```python
from build123d import *

# Parameters (mm, degrees)
F0_R      = 18
F0_R_2    = 5.95
F1_DEPTH  = 4
F2_R      = 18
F2_R_2    = 16
F3_DEPTH  = 1.5
F5_DEPTH  = 1.5
F6_SIZE   = 0.3
F7_COUNT  = 3
F8_R      = 0.75
F9_DEPTH  = 2.5
F10_COUNT = 6
F11_R     = 17
F12_DEPTH = 0.5
F13_SIZE  = 1


with BuildPart() as f1:
    # F0 (on Top) → F1 (new body)
    with BuildSketch(Plane.XY):
        Circle(F0_R)
        Circle(F0_R_2, mode=Mode.SUBTRACT)
    extrude(amount=-F1_DEPTH)

    # F2 (on Top) → F3 (join)
    with BuildSketch(Plane.XY):
        Circle(F2_R)
        Circle(F2_R_2, mode=Mode.SUBTRACT)
    extrude(amount=F3_DEPTH)

    # F4 (on Top) → F5 (join)
    with BuildSketch(Plane.XY):
        with BuildLine():
            Line((-1, -16.7781973636), (1, -16.7781973636))
            Line((1, -16.7781973636), (1, -3.8729833462))
            ThreePointArc((1, -3.8729833462), (0, -4), (-1, -3.8729833462))
            Line((-1, -3.8729833462), (-1, -16.7781973636))
        make_face()
        with BuildLine():
            ThreePointArc((-1, -3.8729833462), (0, -4), (1, -3.8729833462))
            Line((1, -3.8729833462), (1, 3.8729833462))
            ThreePointArc((1, 3.8729833462), (0, 4), (-1, 3.8729833462))
            Line((-1, 3.8729833462), (-1, -3.8729833462))
        make_face()
        with BuildLine():
            Line((1, 3.8729833462), (1, -3.8729833462))
            ThreePointArc((1, -3.8729833462), (3.1622776602, -2.4494897428), (4, 0))
            ThreePointArc((4, 0), (3.1622776602, 2.4494897428), (1, 3.8729833462))
        make_face()
        with BuildLine():
            ThreePointArc((-1, 3.8729833462), (-4, 0), (-1, -3.8729833462))
            Line((-1, -3.8729833462), (-1, 3.8729833462))
        make_face()
        with BuildLine():
            ThreePointArc((-1, 3.8729833462), (0, 4), (1, 3.8729833462))
            Line((1, 3.8729833462), (1, 16.7781973636))
            Line((1, 16.7781973636), (-1, 16.7781973636))
            Line((-1, 16.7781973636), (-1, 3.8729833462))
        make_face()
    extrude(amount=F5_DEPTH)

    # F6
    f6_edges = [f1.edges().sort_by_distance(p)[0] for p in [
        (-18, 0, 1.5),
        (16, 0, 1.5),
        (1, -9.920851, 1.5),
        (4, 0, 1.5),
        (1, 9.920851, 1.5),
        (-16, 0, 1.5),
        (-1, 9.920851, 1.5),
        (-4, 0, 1.5),
        (-1, -9.920851, 1.5),
    ]]
    chamfer(f6_edges, length=F6_SIZE)

    # F7: F1 ×3 about axis
    f7_axis = Axis((0, 0, 0), (0, 0, 1))


with BuildPart() as f1_1:
    add(f1.part)
    for i in range(1, F7_COUNT):
        add(f1.part.rotate(f7_axis, i * 360 / F7_COUNT))

    # F8 (on Top) → F9 (join)
    with BuildSketch(Plane.XY):
        with Locations((0, -16.8108288199)):
            Circle(F8_R)
    extrude(amount=F9_DEPTH)

    # F10: F1 ×6 about axis
    f10_axis = Axis((0, 0, 1.2), (0, 0, -1))


with BuildPart() as f1_2:
    add(f1_1.part)
    for i in range(1, F10_COUNT):
        add(f1_1.part.rotate(f10_axis, i * 360 / F10_COUNT))

    # F11 (on Top) → F12 (join)
    with BuildSketch(Plane.XY):
        Circle(F11_R)
    extrude(amount=F12_DEPTH)

    # F13
    f13_edges = [f1_2.edges().sort_by_distance(p)[0] for p in [
        (-5.95, 0, 0),
    ]]
    chamfer(f13_edges, length=F13_SIZE)


solid = f1_2.part
```
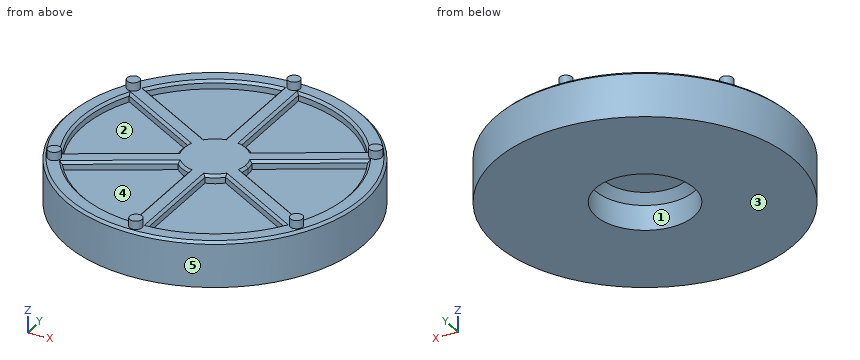
Input: part model. Units: mm. Frame: model coordinates. Face numbers are marked on the shaded views. A direction names the side the tool comes from. Give positions to 0.01 mm unless a question says otherwise; leave off trailing zeros. Write each loop counter-clockwise with the first axis right and the second up, starting at its lowest first coordinate (ties: lowest second). Pieces come first, ordered by that corner, then holes. Notation, with made-up numbers: (18, 85) - (36, 85) arc R13 cw to (36, 95) - close; hole circle Ø2 at (39.25, 83.25). An arc over 180 degrees is marked (long way). Write item = value, one per line. Start each with the question number.
1) Draft query along X for the marked faces 3, 4 and 5. Return one class per face: pulls with the +X half, pulls with the -X half, needs draft (parallel to the pull), parting line crosses it, or undercut.
2) Cut plane A-A (x = 0). Return loops of the section in (y, z).
3) Pin query (flat end, axial travel): pin 1 (3 mm diameter, centred on x = -1.5, y = 1, fed in from -Z); pin 2 (10 mm diameter, centred on x = 4.5, y = 7.5, fed in from +Z); pin 3 (3 mm diameter, centred on y = -6, z = -1, fed in from -X). Return the tip coordinate at first contact, or that it passes through.
4) Material intervals for L1, parallel to Y at x = 0, z = -3.25; L2, parallel to X at y = 3, z = 0.75; L3, parallel to Z at x = 8.5, y = -10, sorted ascending. Write a range as [from, to].
5) Cut plane B-B (z = -1.5). Return loops of the section in (x, y), and give its area (3 significant figures).
6) Reachability of the marked faces 1 and 2 from +Z, -Z, +X, -X, +Y, -Y: full face, straight path, thin tool, end or side. Return the list, or none.
Answers follow:
q1.face_3 = needs draft
q1.face_4 = undercut
q1.face_5 = parting line crosses it
q2.outline = (-18, -4) - (-5.95, -4) - (-5.95, -1) - (-4.95, 0) - (4.95, 0) - (5.95, -1) - (5.95, -4) - (18, -4) - (18, 1.2) - (17.7, 1.5) - (17.56, 1.5) - (17.56, 2.5) - (16.06, 2.5) - (16.06, 1.5) - (-16.06, 1.5) - (-16.06, 2.5) - (-17.56, 2.5) - (-17.56, 1.5) - (-17.7, 1.5) - (-18, 1.2) - close
q3.pin_1 = 0
q3.pin_2 = 1.5
q3.pin_3 = -17.43
q4.L1 = [-18, -5.95], [5.95, 18]
q4.L2 = [-17.75, -15.72], [-7.2, -3.2], [-2.65, 2.65], [3.2, 7.2], [15.72, 17.75]
q4.L3 = [-4, 0.5]
q5.outline = circle Ø36 at (0, 0); hole circle Ø11.9 at (0, 0)
q5.area = 907 mm^2
q6.face_1 = -Z
q6.face_2 = +Z
